The model under review builds one solid part; all positions refer to its coordinate system, in mm. Coordinates: 2 decimals unless noted, no trailing zeros. Loops run counter-clockwise (first coordinate to the right, second up) from the corner with the lowest first, then second, coordinate; pieces in that order, holes last. Notation, with made-up numbers: M 55,64.25 L 110,64.25 A22 cw 110,75.25 Z; hole C 57.5,87.5 d10. An arc over 180 degrees is marked long. Use one line per item in the form item = value.
Autodesk Inventor part; units mm, degrees
ref_plane "YZ Plane" through (0, 0, 0) normal (1, 0, 0) x (0, 1, 0)
ref_plane "XZ Plane" through (0, 0, 0) normal (0, 1, 0) x (-1, 0, 0)
ref_plane "XY Plane" through (0, 0, 0) normal (0, 0, 1) x (1, 0, 0)
sketch "Sketch1" plane through (0, 0, 0) normal (0, 1, 0) x (-1, 0, 0)
  line L0 (17.2372, 12) -> (17.2372, 28) construction
  line L1 (14.9628, 12) -> (17.2372, 12) construction
  line L2 (14.9628, 12) -> (14.9628, 28) construction
  line L3 (17.2372, 28) -> (14.9628, 28) construction
  line L4 (14.2372, 12) -> (14.2372, 28) construction
  line L5 (11.9628, 12) -> (14.2372, 12) construction
  line L6 (11.9628, 12) -> (11.9628, 28) construction
  line L7 (14.2372, 28) -> (11.9628, 28) construction
  line L8 (20.2372, 28) -> (17.9628, 28) construction
  line L9 (20.2372, 12) -> (20.2372, 28) construction
  line L10 (17.9628, 12) -> (20.2372, 12) construction
  line L11 (17.9628, 12) -> (17.9628, 28) construction
  line L12 (11.2372, 12) -> (11.2372, 28) construction
  line L13 (8.9628, 12) -> (11.2372, 12) construction
  line L14 (8.9628, 12) -> (8.9628, 28) construction
  line L15 (11.2372, 28) -> (8.9628, 28) construction
  line L16 (23.2372, 28) -> (20.9628, 28) construction
  line L17 (23.2372, 12) -> (23.2372, 28) construction
  line L18 (20.9628, 12) -> (23.2372, 12) construction
  line L19 (20.9628, 12) -> (20.9628, 28) construction
  line L20 (8.2372, 12) -> (8.2372, 28) construction
  line L21 (5.9628, 12) -> (8.2372, 12) construction
  line L22 (5.9628, 12) -> (5.9628, 28) construction
  line L23 (8.2372, 28) -> (5.9628, 28) construction
  line L24 (26.2372, 28) -> (23.9628, 28) construction
  line L25 (26.2372, 12) -> (26.2372, 28) construction
  line L26 (23.9628, 12) -> (26.2372, 12) construction
  line L27 (23.9628, 12) -> (23.9628, 28) construction
  line L28 (5.2372, 12) -> (5.2372, 28) construction
  line L29 (2.9628, 12) -> (5.2372, 12) construction
  line L30 (2.9628, 12) -> (2.9628, 28) construction
  line L31 (5.2372, 28) -> (2.9628, 28) construction
  line L32 (29.2372, 28) -> (26.9628, 28) construction
  line L33 (29.2372, 12) -> (29.2372, 28) construction
  line L34 (26.9628, 12) -> (29.2372, 12) construction
  line L35 (26.9628, 12) -> (26.9628, 28) construction
  line L36 (2.2372, 12) -> (2.2372, 28) construction
  line L37 (0, 12) -> (2.2372, 12) construction
  line L38 (0, 0) -> (0, 28)
  line L39 (34.1, 0) -> (0, 0)
  line L40 (34.1, 28) -> (34.1, 0)
  line L41 (32.9628, 12) -> (34.1, 12) construction
  line L42 (32.9628, 12) -> (32.9628, 28) construction
  line L43 (34.1, 28) -> (32.9628, 28) construction
  line L44 (34.1, 40) -> (34.1, 28)
  line L45 (0, 40) -> (34.1, 40)
  line L46 (0, 28) -> (0, 40)
  line L47 (2.2372, 28) -> (0, 28) construction
  circle A0 centre (7.05, 34) radius 2.6
  circle A1 centre (27.05, 34) radius 2.6
  circle A2 centre (27.05, 6) radius 2.6
  circle A3 centre (7.05, 6) radius 2.6
  line L48 (32.2372, 28) -> (29.9628, 28) construction
  line L49 (32.2372, 12) -> (32.2372, 28) construction
  line L50 (29.9628, 12) -> (32.2372, 12) construction
  line L51 (29.9628, 12) -> (29.9628, 28) construction
extrude "Extrusion1" add sketch "Sketch1" along normal blind 3.5
properties part number "Y Axis Belt Adjustable Top"
1. Add section B-B (z = 34). State the section outline as (x, y) points.
Response values:
outline = M -34.1,0 L -29.65,0 L -29.65,3.5 L -34.1,3.5 Z; M -24.45,0 L -9.65,0 L -9.65,3.5 L -24.45,3.5 Z; M -4.45,0 L 0,0 L 0,3.5 L -4.45,3.5 Z
2. Add section C-C (x = -27.05). State the section outline as (y, z) points.
Response values:
outline = M 0,0 L 3.5,0 L 3.5,3.4 L 0,3.4 Z; M 0,8.6 L 3.5,8.6 L 3.5,31.4 L 0,31.4 Z; M 0,36.6 L 3.5,36.6 L 3.5,40 L 0,40 Z
3. Wall thickness on line 1 along Z through (x, y) = (-7.05, 1); line 2 along X through (y, z) = (1.45, 35); line 3 along Z through (x, y) = (-6.5, 0.2): over which ranges is each line inside the solid? List them lowest first. Write a range as from..to.
Response values:
line_1 = 0..3.4, 8.6..31.4, 36.6..40
line_2 = -34.1..-29.45, -24.65..-9.45, -4.65..0
line_3 = 0..3.46, 8.54..31.46, 36.54..40
4. Add section A-A (y = 3.05). State the section outline as (x, z) points.
Response values:
outline = M -34.1,0 L 0,0 L 0,40 L -34.1,40 Z; hole C -27.05,6 d5.2; hole C -27.05,34 d5.2; hole C -7.05,6 d5.2; hole C -7.05,34 d5.2
5. The part is to be moulded in two halves that separate along X. For faces 1 (the face through (-26.712, 1.726, 31.422)), 2 (the face through (0, 2, 20)), 3 (the face through (-17, 3.5, 20)), say which applies: pulls with the +X half, pulls with the -X half, needs draft (parallel to the pull), parting line crosses it, or undercut.
Response values:
face_1 = undercut
face_2 = pulls with the +X half
face_3 = needs draft
